Could you check a few things on this model? Use its own coordinates, in mm. A direction names the side the tool comes from. Coordinates: 2 decimals unless noted, no trailing zeros. Write each loop counter-clockwise with the first axis right and the second up, starting at its lowest first coordinate (ties: lowest second). Pieces come first, ordered by that corner, then holes.
Item 1: I want a section at A-A on y = 0. Please give me the cut outline in (x, z).
Item 2: I want a section at B-B on y = 41.5. Please give me the cut outline in (x, z), then the cut area to 3 significant figures.
Item 3: If I drill on probe 1 along Y at (x, z) = (0.8, 0); probe 2 along Y at (x, z) = (-4.75, 11.5); probe 3 along Y at (x, z) = (2.5, 11.5), over which ranges is the centre line in solid material (lowest first)?
Item 4: Which directions (+Z, -Z, +X, -X, +Y, -Y) give clear straight access to the entire face, cutting with the end or side of a thin tool? Please do faces 4 (the flat face through (-0.493, -45.632, 48.095)), 5 (the flat face through (-4.5, -35, 54)), 6 (the flat face through (-0.493, -18.836, -63.567)), 7 (the flat face through (-0.81, -30.9, 53.58)).
Item 5: I want a section at D-D on z = 68.5. Please give me the cut outline in (x, y), then the cut area to 3 significant figures.
Item 6: For P1, Ø7, axis at x = -4, z = 4.5, coming from the -Y side; P2, Ø4, axis at x = -6.5, y = 66.5, coming from the -Z side; P3, Ø4, axis at x = -1.5, y = -21, coming from the +Z side, each with a flat end and sliding along its axis, tell me the tip position at first contact or that it passes through.
Item 7: I want a section at C-C on z = -14.5. Please give me the cut outline in (x, y).
Item 8: Thinking about a two-plate mould opening in Z: for faces 1 (the flat face through (-0.8, 61.8, -0.029)), 2 (the flat face through (3, -35, -35)), 3 (the cylindrical face through (1.521, -38.768, 36.683)), which applies, +Z half, -Z half, draft (parallel to the pull), parting line (faces both ways), or undercut?
from build123d import *

# Parameters (mm, degrees)
SKETCH1_R           = 81
SKETCH1_R_2         = 44.800813008
BOSS_EXTRUDE1_DEPTH = 3
SKETCH2_R           = 2
CUT_EXTRUDE1_DEPTH  = 3
CIRPATTERN1_COUNT   = 8
SKETCH3_W           = 15.5
SKETCH3_H           = 10.25
BOSS_EXTRUDE2_DEPTH = 1
SKETCH4_W           = 12
SKETCH4_H           = 1
BOSS_EXTRUDE3_DEPTH = 9
SKETCH5_W           = 3.5
SKETCH5_H           = 2
BOSS_EXTRUDE4_DEPTH = 9
CIRPATTERN5_COUNT   = 3


with BuildPart() as part:
    # Sketch1 → Boss-Extrude1 (new body)
    with BuildSketch(Plane(origin=(0, 0, 0), x_dir=(0, 0, -1), z_dir=(1, 0, 0))):
        Circle(SKETCH1_R)
        Circle(SKETCH1_R_2, mode=Mode.SUBTRACT)
    extrude(amount=BOSS_EXTRUDE1_DEPTH)

    # Sketch2 → Cut-Extrude1 (cut)
    with BuildSketch(Plane(origin=(3, 0, 0), x_dir=(0, 0, -1), z_dir=(1, 0, 0))):
        with Locations((0, 52)):
            Circle(SKETCH2_R)
    cut_extrude1 = extrude(amount=-CUT_EXTRUDE1_DEPTH, mode=Mode.SUBTRACT)

    # CirPattern1: Cut-Extrude1 ×8 about axis
    cirpattern1_axis = Axis((0, 0, 0), (1, 0, 0))
    for i in range(1, CIRPATTERN1_COUNT):
        add(cut_extrude1.rotate(cirpattern1_axis, i * 360 / CIRPATTERN1_COUNT), mode=Mode.SUBTRACT)

    # Sketch3 → Boss-Extrude2 (add)
    with BuildSketch(Plane(origin=(0, 0, 0), x_dir=(0, 0, -1), z_dir=(1, 0, 0))):
        with Locations((-7.721207901, 64.539778033)):
            Rectangle(SKETCH3_W, SKETCH3_H)
    boss_extrude2 = extrude(amount=-BOSS_EXTRUDE2_DEPTH)

    # Sketch4 → Boss-Extrude3 (add)
    with BuildSketch(Plane(origin=(0, 0, 0), x_dir=(0, 0, -1), z_dir=(1, 0, 0))):
        with Locations((-5.971207901, 59.379009095)):
            Rectangle(SKETCH4_W, SKETCH4_H)
    boss_extrude3 = extrude(amount=-BOSS_EXTRUDE3_DEPTH)

    # Sketch5 → Boss-Extrude4 (add)
    with BuildSketch(Plane(origin=(0, 59.879009095, 0), x_dir=(1, 0, 0), z_dir=(0, 1, 0))):
        with Locations((-6.25, -3.398209268)):
            Rectangle(SKETCH5_W, SKETCH5_H)
    boss_extrude4 = extrude(amount=BOSS_EXTRUDE4_DEPTH)

    # CirPattern5: Boss-Extrude2, Boss-Extrude3, Boss-Extrude4 ×3 about axis
    cirpattern5_axis = Axis((0, 0, 0), (1, 0, 0))
    add([boss_extrude2.rotate(cirpattern5_axis, i * 360 / CIRPATTERN5_COUNT) for i in range(1, CIRPATTERN5_COUNT)])
    add([boss_extrude3.rotate(cirpattern5_axis, i * 360 / CIRPATTERN5_COUNT) for i in range(1, CIRPATTERN5_COUNT)])
    add([boss_extrude4.rotate(cirpattern5_axis, i * 360 / CIRPATTERN5_COUNT) for i in range(1, CIRPATTERN5_COUNT)])


solid = part.part
Response values:
1. outline: (0, -81) - (3, -81) - (3, -54) - (0, -54) - close; (0, -50) - (3, -50) - (3, -44.8) - (0, -44.8) - close; (0, 44.8) - (3, 44.8) - (3, 50) - (0, 50) - close; (0, 54) - (3, 54) - (3, 81) - (0, 81) - close
2. outline: (0, -69.56) - (3, -69.56) - (3, -16.88) - (0, -16.88) - close; (0, 16.88) - (3, 16.88) - (3, 69.56) - (0, 69.56) - close
2. area: 316 mm2
3. probe 1: y = -81 to -54, -50 to -44.8, 44.8 to 50, 54 to 81
3. probe 2: y = 58.88 to 59.88
3. probe 3: y = -80.18 to -43.3, 43.3 to 80.18
4. face 4: -Z, -X, -Y
4. face 5: +Z, -Y
4. face 6: -Z, -X, +Y
4. face 7: +Z, -X, +Y
5. outline: (0, -43.23) - (3, -43.23) - (3, 43.23) - (0, 43.23) - close
5. area: 259 mm2
6. P1: stops at y = 58.88
6. P2: stops at z = 2.4
6. P3: stops at z = 78.57
7. outline: (0, -79.69) - (3, -79.69) - (3, -42.39) - (0, -42.39) - close; (0, 42.39) - (3, 42.39) - (3, 79.69) - (0, 79.69) - close
8. face 1: -Z half
8. face 2: draft
8. face 3: undercut
